Read the model definition and answer for the solid it produces. Units are mm, in the model's axes. A direction names the side the tool comes from. Give positions to 0.01 mm unless a question says otherwise; leave off trailing zeros. Order: outer loops, then holes, each group sorted by start corner. A loop starts at its lowest first (then second) coordinate and runs counter-clockwise, first axis right, second up. Notation, with made-up numbers: (87, 71) -> (137, 71) arc R16 cw to (137, 93) -> close; hole circle Ø6 at (76.5, 70.25). An arc over 180 degrees is marked (long way). One line per item, written item: value. Start each with the question number.
from build123d import *

# Parameters (mm, degrees)
F1_DEPTH = 50
F2_R     = 2.05
F3_DEPTH = 15
F5_R     = 2
F6_DEPTH = 62.001
F5_R_2   = 2.6
F7_DEPTH = 5
F9_DEPTH = 100


with BuildPart() as f1:
    # F0 (on Top) → F1 (new body)
    with BuildSketch(Plane.XY):
        with BuildLine():
            ThreePointArc((34.409301, -2.5), (-25.26361, -23.49468), (0, 34.5))
            Line((0, 34.5), (0, 54.5))
            Line((0, 54.5), (-40, 54.5))
            Line((-40, 54.5), (-40, 39.5))
            Line((-40, 39.5), (-34.423829, 39.5))
            ThreePointArc((-34.423829, 39.5), (-27.548225, 34.996008), (-28.930665, 26.893617))
            ThreePointArc((-28.930665, 26.893617), (-19.51791, -34.340955), (37.909626, -11.095506))
            ThreePointArc((37.909626, -11.095506), (39.710186, -8.498596), (42.708313, -7.5))
            Line((42.708313, -7.5), (54.5, -7.5))
            Line((54.5, -7.5), (54.5, -2.5))
            Line((54.5, -2.5), (34.409301, -2.5))
        make_face()
        with BuildLine():
            ThreePointArc((0, 34.5), (23.49468, 25.26361), (34.409301, 2.5))
            Line((34.409301, 2.5), (54.5, 2.5))
            Line((54.5, 2.5), (54.5, 7.5))
            Line((54.5, 7.5), (54.5, 12.5))
            Line((54.5, 12.5), (40.914545, 12.5))
            ThreePointArc((40.914545, 12.5), (38.16059, 13.326784), (36.317405, 15.533708))
            ThreePointArc((36.317405, 15.533708), (33.114793, 21.532776), (28.930665, 26.893617))
            ThreePointArc((28.930665, 26.893617), (27.548225, 34.996008), (34.423829, 39.5))
            Line((34.423829, 39.5), (40, 39.5))
            Line((40, 39.5), (40, 54.5))
            Line((40, 54.5), (0, 54.5))
            Line((0, 54.5), (0, 34.5))
        make_face()
    extrude(amount=F1_DEPTH)

    # F2 (on face) → F3 (cut)
    with BuildSketch(Plane(origin=(0, 54.5, 0), x_dir=(-1, 0, 0), z_dir=(0, 1, 0))):
        with Locations((-30, 10)):
            Circle(F2_R)
        with Locations((-30, 40)):
            Circle(F2_R)
        with Locations((30, 40)):
            Circle(F2_R)
        with Locations((30, 10)):
            Circle(F2_R)
    extrude(amount=-F3_DEPTH, mode=Mode.SUBTRACT)

    # F5 (on face) → F6 (cut, through all)
    with BuildSketch(Plane.XZ.offset(7.5)):
        with Locations((48.604157, 11.25)):
            Circle(F5_R)
        with Locations((48.604157, 38.75)):
            Circle(F5_R)
    extrude(amount=-F6_DEPTH, mode=Mode.SUBTRACT)

    # F5 (on face) → F7 (cut, through all)
    with BuildSketch(Plane.XZ.offset(7.5)):
        with Locations((48.604157, 11.25)):
            Circle(F5_R_2)
        with Locations((48.604157, 11.25)):
            Circle(F5_R, mode=Mode.SUBTRACT)
        with Locations((48.604157, 38.75)):
            Circle(F5_R_2)
        with Locations((48.604157, 38.75)):
            Circle(F5_R, mode=Mode.SUBTRACT)
    extrude(amount=-F7_DEPTH, mode=Mode.SUBTRACT)

    # F8 (on Right) → F9 (cut, symmetric)
    with BuildSketch(Plane.YZ):
        with BuildLine():
            ThreePointArc((-2.5, 22.5), (0, 25), (-2.5, 27.5))
            Line((-2.5, 27.5), (-48.95404, 27.5))
            ThreePointArc((-48.95404, 27.5), (-51.45404, 25), (-48.95404, 22.5))
            Line((-48.95404, 22.5), (-2.5, 22.5))
        make_face()
    extrude(amount=F9_DEPTH, both=True, mode=Mode.SUBTRACT)


solid = f1.part
Item 1: For a pull along Y with two mould halves and no side action, classify faces 1 (the flat face through (49, -7.5, 36)), 2 (the cylindrical face through (27.5, 34.88, 24.65)), 3 (the cylindrical face through (49.8, -5.04, 36.44)), 4 (the flat face through (-37, 39.5, 25)) as +Y half, -Y half, draft (parallel to the pull), parting line (faces both ways), or undercut.
Item 2: Find the intervals of material crossed by line 1 (Z direction, x = -30, y = 46.75); line 2 (Y direction, x = 30, z = 32); line 3 (Y direction, x = 30, z = 38.5), in increasing order. Write a range as from..to.
Item 3: Find section B-B on y = -15.5. Write down the section's boundary in (x, z), then the cut area to 3 significant figures.
Item 4: Find section A-A on x = 44. Write down the section's boundary in (y, z).
Item 5: Find section D-D on y = 21.5. Write down the section's boundary in (x, z).
Item 6: A tool of negligible diameter and unlimited length cuts with its end or side. For faces 5 (the flat face through (15, -33, 22.5)), 6 (the flat face through (30, 39.5, 40)), 7 (the cylindrical face through (50.51, 7.43, 11.85)), 8 (the flat face through (47, -7.5, 9)), 9 (the flat face through (45, -2.5, 39)), from which of +Z, -Z, +X, -X, +Y, -Y can it reach the whole face along a straight path? Write none if from no direction.
Item 7: Find section C-C on y = 6. Write down the section's boundary in (x, z), then the cut area to 3 significant figures.
Item 8: Flat-ended cylindrical pins translate along their axes: pin 1 (2.5 mm diameter, centred on x = 30, z = 10, fed in from +Y); pin 2 (5 mm diameter, centred on y = -20.5, z = 6, fed in from -X); pin 3 (1 mm diameter, centred on y = 16, z = 15, fed in from +X). Find the tip coordinate at first contact, or state that the pin passes through.
Checks:
1. face 1: -Y half
1. face 2: undercut
1. face 3: draft
1. face 4: undercut
2. line 1: 0..7.95, 12.05..37.95, 42.05..50
2. line 2: -25.7..-17.04, 17.04..25.7, 38.06..54.5
2. line 3: -25.7..-17.04, 17.04..25.7, 38.06..39.5
3. outline: (-36.33, 0) -> (-30.82, 0) -> (-30.82, 22.5) -> (-36.33, 22.5) -> close; (-36.33, 27.5) -> (-30.82, 27.5) -> (-30.82, 50) -> (-36.33, 50) -> close; (30.82, 0) -> (36.33, 0) -> (36.33, 22.5) -> (30.82, 22.5) -> close; (30.82, 27.5) -> (36.33, 27.5) -> (36.33, 50) -> (30.82, 50) -> close
3. area: 496 mm2
4. outline: (-7.5, 0) -> (-2.5, 0) -> (-2.5, 22.5) -> (-7.5, 22.5) -> close; (-7.5, 27.5) -> (-2.5, 27.5) -> (-2.5, 50) -> (-7.5, 50) -> close; (2.5, 0) -> (12.5, 0) -> (12.5, 50) -> (2.5, 50) -> close
5. outline: (-33.14, 0) -> (-26.98, 0) -> (-26.98, 50) -> (-33.14, 50) -> close; (26.98, 0) -> (33.14, 0) -> (33.14, 50) -> (26.98, 50) -> close
6. face 5: +X, -X, -Y
6. face 6: +Y
6. face 7: +Y, -Y
6. face 8: +Z, -Z, +X, -Y
6. face 9: +Z, -Z, +X
7. outline: (-39.04, 0) -> (-33.97, 0) -> (-33.97, 50) -> (-39.04, 50) -> close; (33.97, 0) -> (54.5, 0) -> (54.5, 50) -> (33.97, 50) -> close; hole circle Ø4 at (48.6, 11.25); hole circle Ø4 at (48.6, 38.75)
7. area: 1,250 mm2
8. pin 1: y = 39.5
8. pin 2: x = -35.16
8. pin 3: x = 36.33
